```python
from build123d import *

# Parameters (mm, degrees)
F0_W     = 30
F0_H     = 20
F1_DEPTH = 4
F2_R     = 2.6
F2_W     = 1.5
F2_H     = 6.5
F3_DEPTH = 4.001
F4_W     = 4
F4_H     = 6
F5_DEPTH = 4


with BuildPart() as f1:
    # F0 (on Top) → F1 (new body)
    with BuildSketch(Plane.XY):
        Rectangle(F0_W, F0_H)
    extrude(amount=F1_DEPTH)

    # F2 (on face) → F3 (cut, through all)
    with BuildSketch(Plane.XY.offset(4)):
        with Locations((7, 0)):
            Circle(F2_R)
        with Locations((-1, 0)):
            Rectangle(F2_W, F2_H)
        with Locations((-7, 0)):
            Rectangle(F2_W, F2_H)
    extrude(amount=-F3_DEPTH, mode=Mode.SUBTRACT)

    # F4 (on face) → F5 (join)
    with BuildSketch(Plane.XY.offset(4)):
        with Locations((-13, 0)):
            Rectangle(F4_W, F4_H)
    extrude(amount=F5_DEPTH)


solid = f1.part
```
Geometry check sheet. Reference: the model listing, model coordinates, mm. A direction names the side the tool comes from. Coordinates: 2 decimals unless noted, no trailing zeros. Order: outer loops, then holes, each group sorted by start corner. A loop starts at its lowest first (then second) coordinate and runs counter-clockwise, first axis right, second up. Notation, with made-up numbers: (68, -11.5) - (83, -11.5) arc R4 cw to (83, -6.5) - close; hole circle Ø5 at (7.25, 9.25). An arc over 180 degrees is marked (long way). Use one line per item in the form item = value.
1. Section check A-A (y = 0). Record the boundary of the cut face in (x, z), then the cut area to 3 significant figures.
Here are the results:
outline = (-15, 0) - (-7.75, 0) - (-7.75, 4) - (-11, 4) - (-11, 8) - (-15, 8) - close; (-6.25, 0) - (-1.75, 0) - (-1.75, 4) - (-6.25, 4) - close; (-0.25, 0) - (4.4, 0) - (4.4, 4) - (-0.25, 4) - close; (9.6, 0) - (15, 0) - (15, 4) - (9.6, 4) - close
area = 103 mm²
2. Section check D-D (y = -7). Record the boundary of the cut face in (x, z).
Here are the results:
outline = (-15, 0) - (15, 0) - (15, 4) - (-15, 4) - close
3. Access from +Z, -Z, +X, -X, +Y, -Y to the whole of each face (thin tool, end or side, straight path). Record for faces 1 (the face through (0, -10, 2)), 2 (the face through (15, 0, 2)), 3 (the face through (-13, 3, 6)), 4 (the face through (-13, -3, 6)), 5 (the face through (-0.25, 0, 2)).
Here are the results:
face_1 = +Z, -Z, +X, -X, -Y
face_2 = +Z, -Z, +X, +Y, -Y
face_3 = +Z, +X, -X, +Y
face_4 = +Z, +X, -X, -Y
face_5 = +Z, -Z
4. Section check C-C (z = 1.25). Record the boundary of the cut face in (x, y), then the cut area to 3 significant figures.
Here are the results:
outline = (-15, -10) - (15, -10) - (15, 10) - (-15, 10) - close; hole (-7.75, -3.25) - (-6.25, -3.25) - (-6.25, 3.25) - (-7.75, 3.25) - close; hole (-1.75, -3.25) - (-0.25, -3.25) - (-0.25, 3.25) - (-1.75, 3.25) - close; hole circle Ø5.2 at (7, 0)
area = 559 mm²
5. Draft check along X on faces 6 (the face through (-13, 0, 8)), 7 (the face through (-7, 3.25, 2)), 8 (the face through (-11, 0, 6)). Enter one of: pulls with the +X half, pulls with the -X half, needs draft (parallel to the pull), parting line crosses it, or undercut.
Here are the results:
face_6 = needs draft
face_7 = undercut
face_8 = pulls with the +X half
6. Section check B-B (x = 7). Record the boundary of the cut face in (y, z).
Here are the results:
outline = (-10, 0) - (-2.6, 0) - (-2.6, 4) - (-10, 4) - close; (2.6, 0) - (10, 0) - (10, 4) - (2.6, 4) - close
7. Scan lines: line 1 (Y direction, x = 7, z = 2.1); line 2 (Z direction, x = -9.25, y = 8.25); line 3 (X direction, y = 1.5, z = 6.5). Record each from-to range of solid material in increasing order.
Here are the results:
line_1 = -10 to -2.6, 2.6 to 10
line_2 = 0 to 4
line_3 = -15 to -11
8. Gauge pin test, flat ends, axial feed: pin 1 (1.2 mm diameter, centred on y = 1, z = 6, fed in from +X); pin 2 (2 mm diameter, centred on x = -14, z = 5.5, fed in from -Y); pin 3 (3 mm diameter, centred on x = -10, z = 6, fed in from +Y); pin 4 (5 mm diameter, centred on x = -0.5, y = -5, fed in from -Z). Record the tip position at first contact, or that the pin passes through.
Here are the results:
pin_1 = -11
pin_2 = -3
pin_3 = 3
pin_4 = 0
